Geometry check sheet. Reference: the model listing, model coordinates, mm. A direction names the side the tool comes from. Round coordinates to 2 decimals unless told otherwise and drop trailing zeros. Write each loop counter-clockwise with the first axis right and the second up, starting at its lowest first coordinate (ties: lowest second). Pieces come first, ordered by that corner, then holes.
Item 1: Cross-section at B-B (z = 0). Enter the section's corners in (x, y).
Item 2: Depth check by flat-ended pin: P1, Ø3, axis at x = -40.5, y = -5, coming from the +Z side; P2, Ø5, axis at x = 65, y = -2.5, coming from the -Z side; P3, Ø4, axis at y = -5, z = 25, coming from the +X side. Enter the tip coordinate at first touch or a pass-through.
Item 3: Draft check along X on faces 1 (the face through (95.38, -6.26, 30.04)), 2 (the face through (-1, 0, -65)), 3 (the face through (1, -6, -63.5)). Enter one of: pulls with the +X half, pulls with the -X half, needs draft (parallel to the pull), parting line crosses it, or undercut.
Item 4: Cross-section at C-C (x = -29). Enter the section's corners in (y, z), then the cut area to 3 significant figures.
Item 5: Scan lines: probe 1 along Z at (x, y) = (0, -10); probe 2 along Z at (x, y) = (-3.5, -2); probe 3 along X at (y, z) = (-3.75, 15). Record each from-to range of solid material in increasing order.
Item 6: Access from +Z, -Z, +X, -X, +Y, -Y to the whole of each face (thin tool, end or side, straight path). Record for faces 4 (the face through (-60.628, -6.261, -60.777)), 5 (the face through (-1, -12.7, -65)).
Item 7: Cross-section at A-A (x = 0). Enter the section's corners in (y, z), then the cut area to 3 significant figures.
Item 8: Cross-section at D-D (y = -2.75). Enter the section's corners in (x, z), then the cut area to 3 significant figures.
from build123d import *

# Parameters (mm, degrees)
F0_R     = 100
F1_DEPTH = 12.7
F2_D     = 10.5


with BuildPart() as f1:
    # F0 (on Front) → F1 (new body)
    with BuildSketch(Plane.XZ):
        Circle(F0_R)
        with BuildLine():
            ThreePointArc((63.5, -53.95), (60.7028697603, -60.7028697603), (53.95, -63.5))
            Line((53.95, -63.5), (-53.95, -63.5))
            ThreePointArc((-53.95, -63.5), (-60.7028697603, -60.7028697603), (-63.5, -53.95))
            Line((-63.5, -53.95), (-63.5, 53.95))
            ThreePointArc((-63.5, 53.95), (-60.7028697603, 60.7028697603), (-53.95, 63.5))
            Line((-53.95, 63.5), (53.95, 63.5))
            ThreePointArc((53.95, 63.5), (60.7028697603, 60.7028697603), (63.5, 53.95))
            Line((63.5, 53.95), (63.5, -53.95))
        make_face(mode=Mode.SUBTRACT)
    extrude(amount=F1_DEPTH)

    # F2 (through all)
    with Locations(Plane(origin=(0, 0, 0), x_dir=(1, 0, 0), z_dir=(0, 1, 0))):
        with Locations((0, -81.754), (81.754, 0), (0, 81.754), (-81.754, 0)):
            Hole(F2_D / 2)


solid = f1.part
Resolved:
1. outline: (-100, -12.7) - (-87, -12.7) - (-87, 0) - (-100, 0) - close; (-76.5, -12.7) - (-63.5, -12.7) - (-63.5, 0) - (-76.5, 0) - close; (63.5, -12.7) - (76.5, -12.7) - (76.5, 0) - (63.5, 0) - close; (87, -12.7) - (100, -12.7) - (100, 0) - (87, 0) - close
2. P1: stops at z = 92.08
2. P2: stops at z = -78.06
2. P3: stops at x = 97.32
3. face 1: parting line crosses it
3. face 2: needs draft
3. face 3: undercut
4. outline: (-12.7, -95.7) - (0, -95.7) - (0, -63.5) - (-12.7, -63.5) - close; (-12.7, 63.5) - (0, 63.5) - (0, 95.7) - (-12.7, 95.7) - close
4. area: 818 mm2
5. probe 1: z = -100 to -87, -76.5 to -63.5, 63.5 to 76.5, 87 to 100
5. probe 2: z = -99.94 to -85.67, -77.84 to -63.5, 63.5 to 77.84, 85.67 to 99.94
5. probe 3: x = -98.87 to -63.5, 63.5 to 98.87
6. face 4: +Y, -Y
6. face 5: +Z, -Z, +X, -X, -Y
7. outline: (-12.7, -100) - (0, -100) - (0, -87) - (-12.7, -87) - close; (-12.7, -76.5) - (0, -76.5) - (0, -63.5) - (-12.7, -63.5) - close; (-12.7, 63.5) - (0, 63.5) - (0, 76.5) - (-12.7, 76.5) - close; (-12.7, 87) - (0, 87) - (0, 100) - (-12.7, 100) - close
7. area: 660 mm2
8. outline: circle Ø200 at (0, 0); hole circle Ø10.5 at (-81.75, 0); hole (-63.5, -53.95) arc R9.55 ccw to (-53.95, -63.5) - (53.95, -63.5) arc R9.55 ccw to (63.5, -53.95) - (63.5, 53.95) arc R9.55 ccw to (53.95, 63.5) - (-53.95, 63.5) arc R9.55 ccw to (-63.5, 53.95) - close; hole circle Ø10.5 at (0, -81.75); hole circle Ø10.5 at (0, 81.75); hole circle Ø10.5 at (81.75, 0)
8. area: 15,000 mm2
